Here's the drawing with two shaded views (mm, measured from the low corner). I have some questions. A direction names the side the tool comes from. Round coordinates to 2 decimals unless told otherwise and drop trailing zeros. Loops run counter-clockwise (first coordinate to the right, second up) from the corner with the lowest first, then second, coordinate; pieces in that order, holes last.
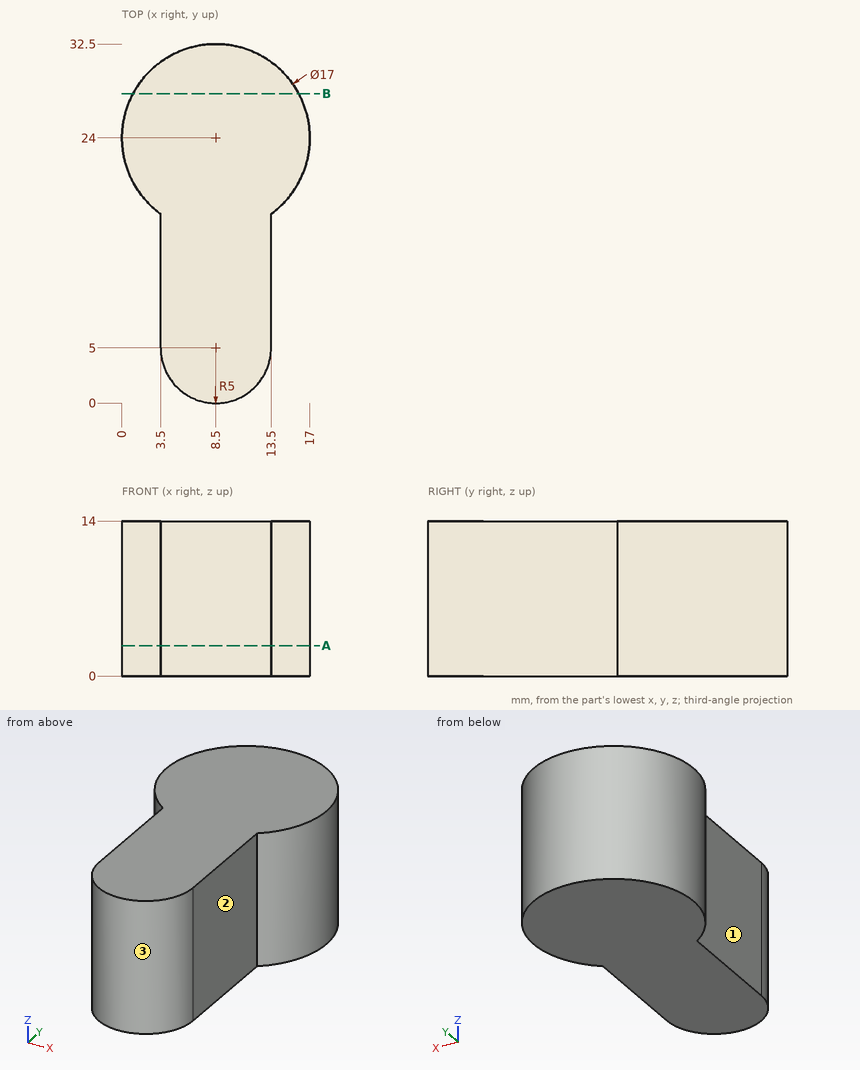
Item 1: If I drill on line 1 along X through (y, z) = (17, 2.75); line 2 along X through (y, z) = (2.5, 8.5); line 3 along Y through (x, z) = (2.75, 11), over which ranges is the centre line in solid material (lowest first)?
Results list:
line 1: x = 3.5 to 13.5
line 2: x = 4.17 to 12.83
line 3: y = 17.74 to 30.26
Item 2: If we section it at A-A, the plane z = 2.75: Please give me the cut outline in (x, y).
Results list:
outline: (3.5, 5) arc R5 ccw to (13.5, 5) - (13.5, 17.13) arc R8.5 ccw (long way) to (3.5, 17.13) - close
Item 3: For the marked faces 1, 2 and 3, which set-ups out of +Z, -Z, +X, -X, +Y, -Y let a thin tool reach every point of the face, with its end or its side?
Results list:
face 1: +Z, -Z, -X, -Y
face 2: +Z, -Z, +X, -Y
face 3: +Z, -Z, -Y
Item 4: If we section it at B-B, the plane y = 28: Please give me the cut outline in (x, z), then the cut area to 3 significant figures.
Results list:
outline: (1, 0) - (16, 0) - (16, 14) - (1, 14) - close
area: 210 mm2
Item 5: Will these pins go through, and if not, where does the flat tip stop? pin 1 (8 mm diameter, centred on y = 24.5, z = 7.5, fed in from -X); pin 2 (1 mm diameter, centred on y = 13.5, z = 5, fed in from +X); pin 3 (5 mm diameter, centred on x = 14, z = 9.5, fed in from -Y); pin 4 (5 mm diameter, centred on x = 2.5, z = 4.5, fed in from -Y).
Results list:
pin 1: stops at x = 0
pin 2: stops at x = 13.5
pin 3: stops at y = 1
pin 4: stops at y = 1.43
